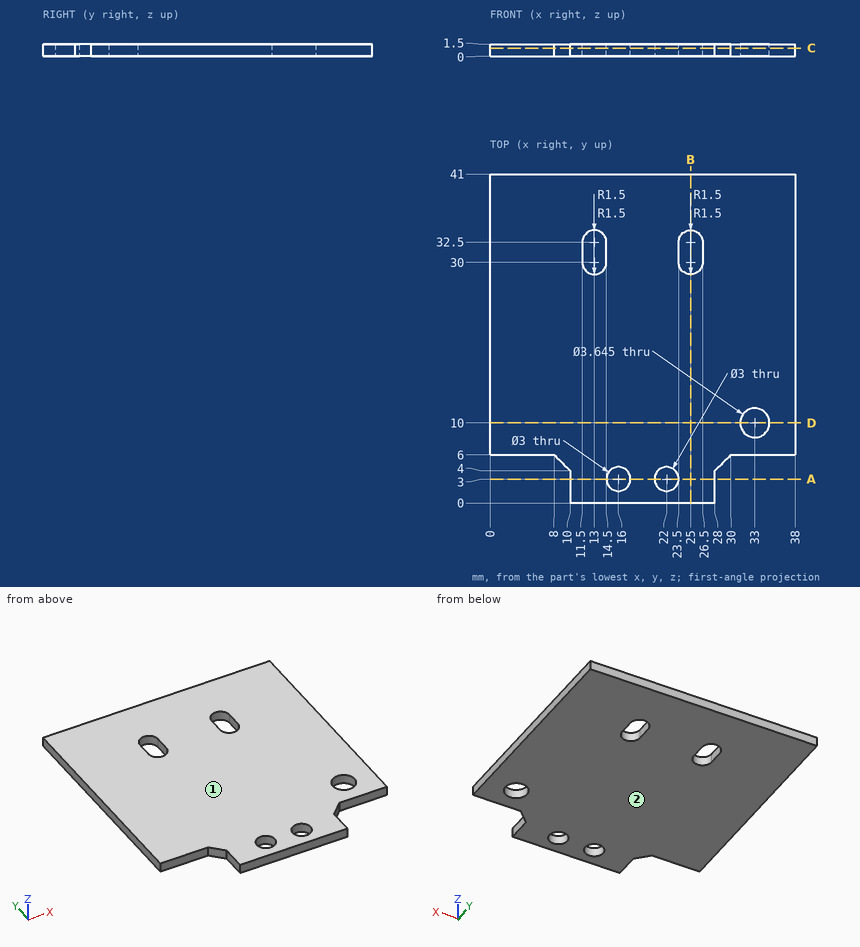
Geometry: see drawing. Coordinates: mm, zero at the bounding-box minimum. Round coordinates to 2 decimals unless told otherwise and drop trailing zeros. Write each loop counter-clockwise with the first axis right and the second up, starting at its lowest first coordinate (ties: lowest second). Pieces come first, ordered by that corner, then holes. Notation, with made-up numbers: M -40,51 L -31,51 A6 cw -31,61 Z; hole C 16.5,41 d2. An arc over 180 degrees is marked long. Answer in a Markdown table with one row per item. Add a question column.
(1) Contact query for flat-ended pins moving along their axis: pin 1 (3.5 mm diameter, centred on x = 22, y = 3, fed in from +Z); pin 2 (0.8 mm diameter, centred on y = 1, z = 1, fed in from +X); pin 3 (0.8 mm diameter, centred on x = 33, z = 1, fed in from -Y). Output: stop coordinate, or through.
(2) Ray query, L1, parallel to Y at x = 33, z = 0.65; L2, parallel to Y at x = 25, z = 1.45; L3, parallel to Y at x = 36.5, z = 0.9. Return the intervals inside material, ascending.
(3) Cut plane C-C, the plane z = 1. Return the cut outline in (x, y) (1 decimal), then the cut area to 3 significant figures.
(4) Cut plane D-D, the plane y = 10. Return the cut outline in (x, z).
(5) Cut plane B-B, the plane x = 25. Return the cut outline in (y, z).
(6) Cut plane A-A, the plane y = 3. Return the cut outline in (x, z), then the cut area to 3 significant figures.
(7) Draft query along Z for the marked faces 1 and 2. Return one class per face: pulls with the +Z half, pulls with the -Z half, needs draft (parallel to the pull), parting line crosses it, or undercut.
Established:
| question | item | result |
|---|---|---|
| 1 | pin 1 | z = 1.5 |
| 1 | pin 2 | x = 28 |
| 1 | pin 3 | y = 6 |
| 2 | L1 | 6 to 8.18, 11.82 to 41 |
| 2 | L2 | 0 to 28.5, 34 to 41 |
| 2 | L3 | 6 to 41 |
| 3 | outline | M 0,6 L 8,6 L 10,4 L 10,0 L 28,0 L 28,4 L 30,6 L 38,6 L 38,41 L 0,41 Z; hole M 11.5,30 A1.5 ccw 14.5,30 L 14.5,32.5 A1.5 ccw 11.5,32.5 Z; hole C 16,3 d3; hole C 22,3 d3; hole M 23.5,30 A1.5 ccw 26.5,30 L 26.5,32.5 A1.5 ccw 23.5,32.5 Z; hole C 33,10 d3.6 |
| 3 | area | 1,390 mm² |
| 4 | outline | M 0,0 L 31.18,0 L 31.18,1.5 L 0,1.5 Z; M 34.82,0 L 38,0 L 38,1.5 L 34.82,1.5 Z |
| 5 | outline | M 0,0 L 28.5,0 L 28.5,1.5 L 0,1.5 Z; M 34,0 L 41,0 L 41,1.5 L 34,1.5 Z |
| 6 | outline | M 10,0 L 14.5,0 L 14.5,1.5 L 10,1.5 Z; M 17.5,0 L 20.5,0 L 20.5,1.5 L 17.5,1.5 Z; M 23.5,0 L 28,0 L 28,1.5 L 23.5,1.5 Z |
| 6 | area | 18.0 mm² |
| 7 | face 1 | pulls with the +Z half |
| 7 | face 2 | pulls with the -Z half |
